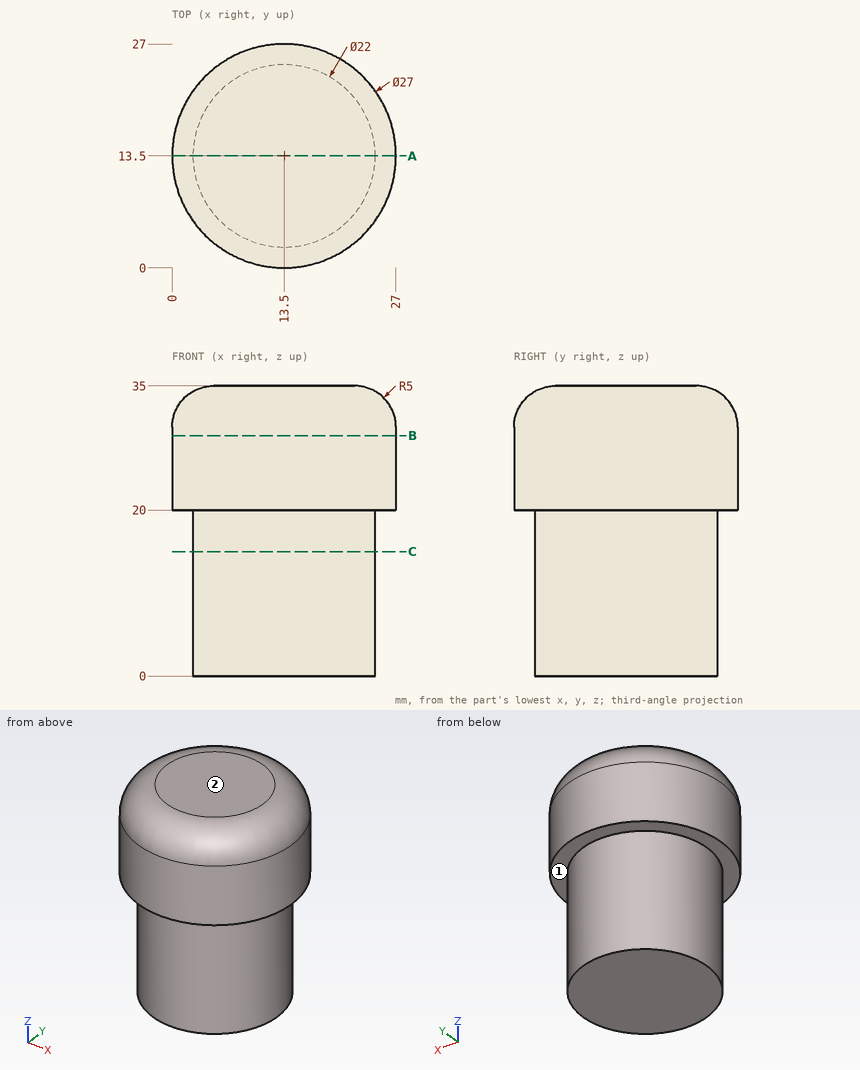
Design review of the part shown in the three views and the two pictorial views. Dimensions are in mm from the part's minimum x, y and z. A direction names the side the tool comes from. Coordinates: 2 decimals unless noted, no trailing zeros. Loops run counter-clockwise (first coordinate to the right, second up) from the corner with the lowest first, then second, coordinate; pieces in that order, holes last. Notation, with made-up numbers: (16.5, 89.5) -> (46.5, 89.5) arc R11 cw to (46.5, 100.5) -> close; hole circle Ø4 at (57, 40). An arc over 180 degrees is marked (long way). Answer as CSV lines item,"result".
Item 1: Take a section at B-B, the plane z = 29. State the section outline as (x, y) points, and give its area (3 significant figures).
Results below:
outline,"circle Ø27 at (13.5, 13.5)"
area,"573 mm2"
Item 2: Take a section at C-C, the plane z = 15. State the section outline as (x, y) points, and give its area (3 significant figures).
Results below:
outline,"circle Ø22 at (13.5, 13.5)"
area,"380 mm2"
Item 3: Insertion check: pin 1 (6 mm diameter, centred on x = 23, z = 20, fed in from -Y); pin 2 (1 mm diameter, centred on x = 17.5, z = 30.5, fed in from -Y); pin 3 (8 mm diameter, centred on y = 7, z = 31, fed in from -X); pin 4 (8 mm diameter, centred on x = 19.5, y = 4, fed in from +Z). Each pin has a flat end and moves straight along its axis. Give the tip position at first contact, or say it passes through.
Results below:
pin 1,"stops at y = 1.67"
pin 2,"stops at y = 0.48"
pin 3,"stops at x = 0.25"
pin 4,"stops at z = 35"
Item 4: Take a section at A-A, the plane y = 13.5. State the section outline as (x, z) points, and give its area (3 significant figures).
Results below:
outline,"(0, 20) -> (2.5, 20) -> (2.5, 0) -> (24.5, 0) -> (24.5, 20) -> (27, 20) -> (27, 30) arc R5 ccw to (22, 35) -> (5, 35) arc R5 ccw to (0, 30) -> close"
area,"834 mm2"
Item 5: Machinability: for the marked faces 1 and 2, which of the approach directions +Z, -Z, +X, -X, +Y, -Y give a long, thin tool a straight path to every point of the face, cutting with its end or side? Answer none if there is none.
Results below:
face 1,"-Z"
face 2,"+Z, +X, -X, +Y, -Y"
Item 6: For L1, parallel to Z at x = 15.5, y = 22; L2, parallel to X at y = 8, z = 28; L3, parallel to X at y = 23.25, z = 2, list the stretches that pass through material, from the lowest coordinate up.
Results below:
L1,"z = 0 to 34.99"
L2,"x = 1.17 to 25.83"
L3,"x = 8.41 to 18.59"
